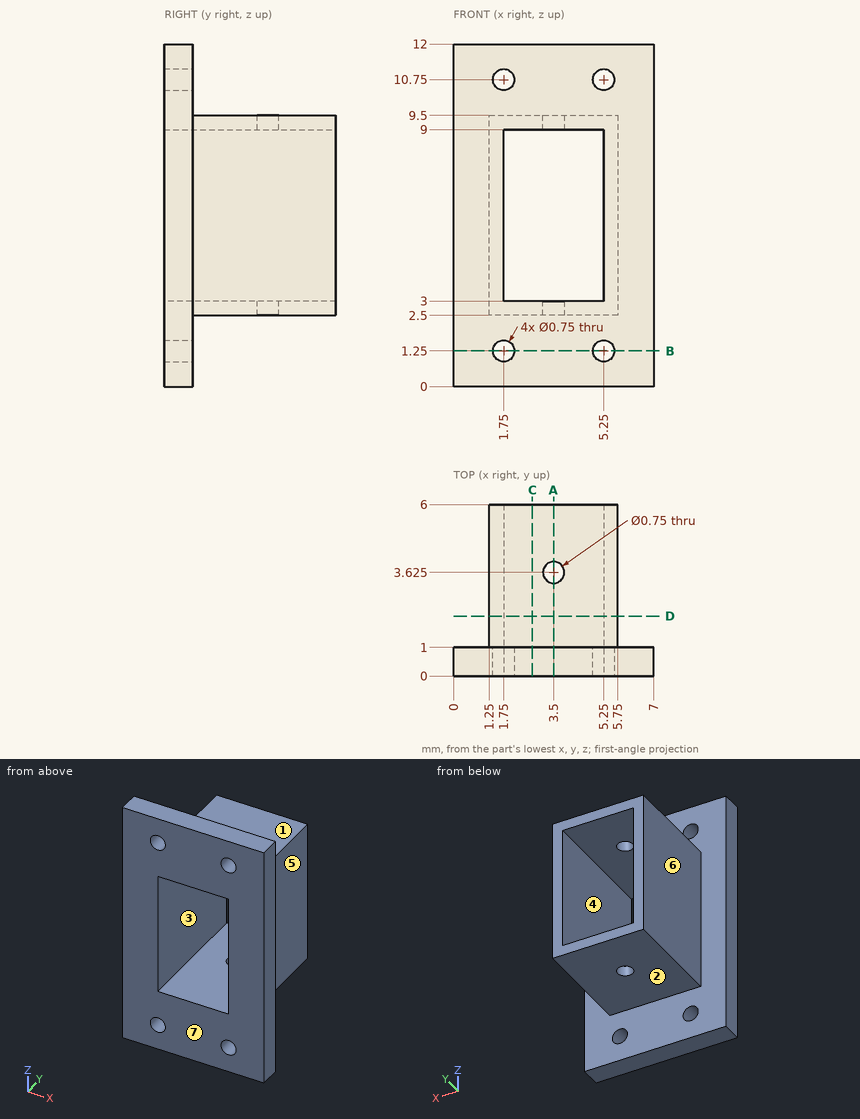
Input: dimensioned drawing with shaded views. Units: mm. Origin: part minimum x, y, z. A direction names the side the tool comes from. Round coordinates to 2 decimals unless told otherwise and drop trailing zeros. Loops run counter-clockwise (first coordinate to the right, second up) from the corner with the lowest first, then second, coordinate; pieces in that order, holes last. Notation, with made-up numbers: M 53,57.5 L 71,57.5 A21 cw 71,81.5 Z; hole C -30,76.5 d2. An arc over 180 degrees is marked long. One line per question, with ' | ' between items.
(1) Material intervals for line 1 along X through (y, z) = (0.55, 10.75) (3 decimals); line 2 along X through (y, z) = (0.65, 6); line 3 along Z through (x, y) = (2.25, 0.9), sorted ascending. Write a range as from..to.
Check result:
line 1: x = 0..1.375, 2.125..4.875, 5.625..7 | line 2: x = 0..1.75, 5.25..7 | line 3: z = 0..3, 9..12
(2) Cut plane D-D on y = 2.1. Return the cut outline in (x, z), plus the area to 3 significant figures.
Check result:
outline: M 1.25,2.5 L 5.75,2.5 L 5.75,9.5 L 1.25,9.5 Z; hole M 1.75,3 L 5.25,3 L 5.25,9 L 1.75,9 Z | area: 10.5 mm2
(3) Contact query for flat-ended pins moving along their axis: P1, Ø3, axis at y = 4, z = 5.5, coming from the +X side; P2, Ø2, axis at x = 3.5, y = 4, coming from the +Z side; P3, Ø1.8, axis at x = 3.5, y = 2.5, coming from the -Z side. Output: stop coordinate, or through.
Check result:
P1: stops at x = 5.75 | P2: stops at z = 9.5 | P3: stops at z = 2.5
(4) Pull-direction query (X, two-part tool) for the marked faces 4, 5, 6 and 7; classes: +X half, -X half, draft (parallel to the pull), parting line (faces both ways), or undercut.
Check result:
face 4: undercut | face 5: +X half | face 6: -X half | face 7: draft
(5) Cut plane A-A on x = 3.5. Return the cut outline in (y, z), plus the area to 4 significant figures.
Check result:
outline: M 0,0 L 1,0 L 1,2.5 L 3.25,2.5 L 3.25,3 L 0,3 Z; M 0,9 L 3.25,9 L 3.25,9.5 L 1,9.5 L 1,12 L 0,12 Z; M 4,2.5 L 6,2.5 L 6,3 L 4,3 Z; M 4,9 L 6,9 L 6,9.5 L 4,9.5 Z | area: 10.25 mm2
(6) Cut plane B-B on z = 1.25. Return the cut outline in (x, y) (3 decimals).
Check result:
outline: M 0,0 L 1.375,0 L 1.375,1 L 0,1 Z; M 2.125,0 L 4.875,0 L 4.875,1 L 2.125,1 Z; M 5.625,0 L 7,0 L 7,1 L 5.625,1 Z
(7) Access query for the marked faces 1, 2 and 3. Directions: +Z, -Z, +X, -X, +Y, -Y. A direction counts if a zero-diameter tool reaches every point of the face in a straight line with its end or side. Return the directions, or none.
Check result:
face 1: +Z, +X, -X, +Y | face 2: -Z, +X, -X, +Y | face 3: +Y, -Y
(8) Cut plane C-C on x = 2.75. Return the cut outline in (y, z), plus the area to 3 significant figures.
Check result:
outline: M 0,0 L 1,0 L 1,2.5 L 6,2.5 L 6,3 L 0,3 Z; M 0,9 L 6,9 L 6,9.5 L 1,9.5 L 1,12 L 0,12 Z | area: 11.0 mm2
